For this review, take the finished solid that the model builds, in its own axes (mm). A direction names the side the tool comes from. Give positions to 0.01 mm unless a question says otherwise; leave off trailing zeros. Order: outer loops, then holes, each group sorted by start corner. A loop starts at its lowest first (then second) coordinate and runs counter-clockwise, first axis right, second up. Notation, with made-up numbers: (78, 13.5) -> (99, 13.5) arc R20 ccw to (99, 22.5) -> close; hole circle Ø3 at (25, 80). An arc over 180 degrees is marked (long way). Return JSON: item names as keys, results as strings. Group by question number.
1) To check wall thickness, follow line 1 along Y through (x, z) = (25, 28); line 2 along X through (y, z) = (-4, 6.5); line 3 along Y through (x, z) = (-29.5, 28). State the ranges of each line that lie inside material, in increasing order.
2) Add section A-A (x = 25.4). Give the boundary of the cut face in (y, z), then the cut area to 3 significant figures.
3) Add section B-B (z = 30). Give the boundary of the cut face in (x, y), then the cut area to 3 significant figures.
4) For faces 4 (the face through (-1, 0, 0)), 5 (the face through (-1, -25.4, 15)), 6 (the face through (-0.419, 28.531, 19.055)), list the 3-axis set-ups (+Z, -Z, +X, -X, +Y, -Y) from which the entire face can be reached by the end or side of a thin tool; tool diameter is ignored.
5) The part is to be moulded in two halves that separate along Y. For faces 1 (the face through (-0.419, -28.531, 19.055)), 2 (the face through (-19.343, 1.907, 18.783)), 3 (the face through (-1, 25.4, 15)), say which applies: released by +Y, released by -Y, zero draft, split by the parting line, or undercut.
6) Insertion check: P1, Ø1, axis at x = -22.5, y = 17.5, coming from the -Z side; P2, Ø10, axis at x = -2, z = 32, coming from the -Y side; P3, Ø5, axis at x = -27.5, z = 20, coming from the -Y side. Each pin has a flat end and moves straight along its axis. Give the tip position at first contact, or say it passes through.
7) Add section C-C (y = 0). Give the boundary of the cut face in (x, z), then the cut area to 3 significant figures.
8) Add section D-D (z = 5). Give the boundary of the cut face in (x, y).
from build123d import *

# Parameters (mm, degrees)
F0_W     = 76.2
F0_H     = 50.8
F0_R     = 6.35
F1_DEPTH = 38.1
F3_DEPTH = 50.801
F4_DEPTH = 6.35


with BuildPart() as f1:
    # F0 (on Top) → F1 (new body)
    with BuildSketch(Plane.XY):
        Rectangle(F0_W, F0_H)
        with Locations((-25.4, 0)):
            Circle(F0_R, mode=Mode.SUBTRACT)
        with Locations((25.4, 0)):
            Circle(F0_R, mode=Mode.SUBTRACT)
    extrude(amount=F1_DEPTH)

    # F2 (on face) → F3 (cut, through all)
    with BuildSketch(Plane.XZ.offset(25.4)):
        with BuildLine():
            ThreePointArc((-12.7, 38.1), (0, 25.4), (12.7, 38.1))
            Line((12.7, 38.1), (-12.7, 38.1))
        make_face()
    extrude(amount=-F3_DEPTH, mode=Mode.SUBTRACT)

    # F2 (on face) → F4 (join)
    with BuildSketch(Plane.XZ.offset(25.4)):
        with BuildLine():
            ThreePointArc((-19.05, 38.1), (0, 19.05), (19.05, 38.1))
            Line((19.05, 38.1), (12.7, 38.1))
            ThreePointArc((12.7, 38.1), (0, 25.4), (-12.7, 38.1))
            Line((-12.7, 38.1), (-19.05, 38.1))
        make_face()
    extrude(amount=F4_DEPTH)

    # F5: F1 across plane


with BuildPart() as f1_1:
    add(f1.part)
    add(f1.part.mirror(Plane.XZ))


solid = f1_1.part
Evaluation:
{
 "1": {"line 1": "-25.4 to -6.34, 6.34 to 25.4", "line 2": "-38.1 to -30.33, -20.47 to 20.47, 30.33 to 38.1", "line 3": "-25.4 to -4.85, 4.85 to 25.4"},
 "2": {"outline": "(-25.4, 0) -> (-6.35, 0) -> (-6.35, 38.1) -> (-25.4, 38.1) -> close; (6.35, 0) -> (25.4, 0) -> (25.4, 38.1) -> (6.35, 38.1) -> close", "area": "1,450 mm^2"},
 "3": {"outline": "(-38.1, -25.4) -> (-17.24, -25.4) -> (-17.24, -31.75) -> (-9.78, -31.75) -> (-9.78, 31.75) -> (-17.24, 31.75) -> (-17.24, 25.4) -> (-38.1, 25.4) -> close; (9.78, -31.75) -> (17.24, -31.75) -> (17.24, -25.4) -> (38.1, -25.4) -> (38.1, 25.4) -> (17.24, 25.4) -> (17.24, 31.75) -> (9.78, 31.75) -> close; hole circle Ø12.7 at (-25.4, 0); hole circle Ø12.7 at (25.4, 0)", "area": "2,810 mm^2"},
 "4": {"face 4": "-Z, +X, -X, +Y, -Y", "face 5": "-Z, -Y", "face 6": "-Z, +Y"},
 "5": {"face 1": "zero draft", "face 2": "undercut", "face 3": "released by +Y"},
 "6": {"P1": "z = 0", "P2": "through", "P3": "y = -25.4"},
 "7": {"outline": "(-38.1, 0) -> (-31.75, 0) -> (-31.75, 38.1) -> (-38.1, 38.1) -> close; (-19.05, 0) -> (19.05, 0) -> (19.05, 38.1) -> (12.7, 38.1) arc R12.7 cw to (-12.7, 38.1) -> (-19.05, 38.1) -> close; (31.75, 0) -> (38.1, 0) -> (38.1, 38.1) -> (31.75, 38.1) -> close", "area": "1,680 mm^2"},
 "8": {"outline": "(-38.1, -25.4) -> (38.1, -25.4) -> (38.1, 25.4) -> (-38.1, 25.4) -> close; hole circle Ø12.7 at (-25.4, 0); hole circle Ø12.7 at (25.4, 0)"}
}
